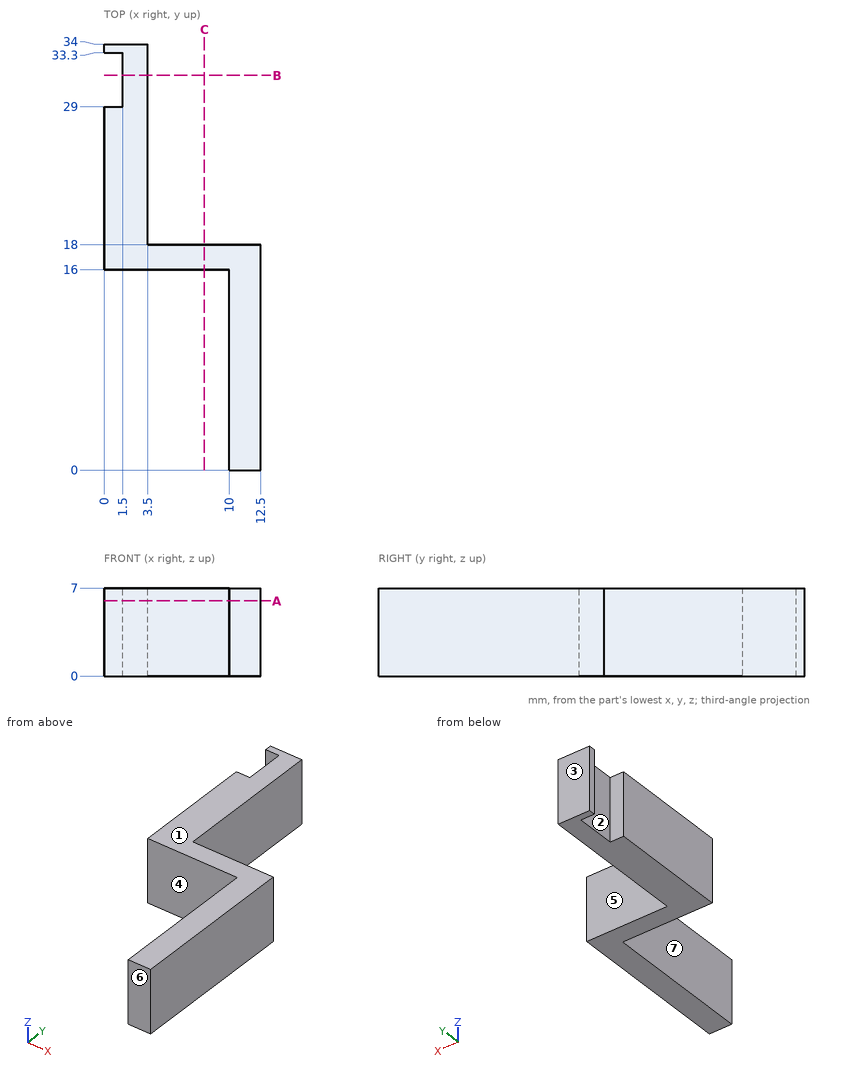
Can you work these out from the drawing? Everything is in mm from the part's minimum corner. A direction names the side the tool comes from. Round coordinates to 2 decimals unless told otherwise and drop trailing zeros. Write each loop counter-clockwise with the first axis right and the second up, starting at its lowest first coordinate (ties: lowest second). Pieces come first, ordered by that corner, then holes. Notation, with made-up numbers: M 63,28.25 L 119,28.25 A17 cw 119,36.25 Z; hole C -38,81.5 d2. An arc over 180 degrees is marked long. Use a Markdown table: item, result.
Item 1: I want a section at B-B (y = 31.5). List the corners of the cut face in (x, z) for me, and give its area (3 significant figures).
Found:
| item | result |
|---|---|
| outline | M 1.5,0 L 3.5,0 L 3.5,7 L 1.5,7 Z |
| area | 14.0 mm2 |
Item 2: I want a section at C-C (x = 8). List the corners of the cut face in (y, z) for me, and give its area (3 significant figures).
Found:
| item | result |
|---|---|
| outline | M 16,0 L 18,0 L 18,7 L 16,7 Z |
| area | 14.0 mm2 |
Item 3: For pin 1 Ø3.5 at (x, z) = (6.5, 3) entering from -Y; pin 2 Ø3.5 at (y, z) = (8, 2) entering from -X; pin 3 Ø3.5 at (x, z) = (8.5, 5) entering from +Y; pin 4 Ø4 at (x, y) = (7, 11) entering from -Z, each with a flat end and sliding along its axis, tell me the tip position at first contact or that it passes through.
Found:
| item | result |
|---|---|
| pin 1 | stops at y = 16 |
| pin 2 | stops at x = 10 |
| pin 3 | stops at y = 18 |
| pin 4 | passes through |
Item 4: We'd pull the mould along Y, two halves only. Please class the marked faces 1, 2, 3 and 4: released by +Y, released by -Y, zero draft, split by the parting line, or undercut.
Found:
| item | result |
|---|---|
| face 1 | zero draft |
| face 2 | undercut |
| face 3 | released by +Y |
| face 4 | released by -Y |
Item 5: I want a section at A-A (z = 6). List the corners of the cut face in (x, y) for me.
Found:
| item | result |
|---|---|
| outline | M 0,16 L 10,16 L 10,0 L 12.5,0 L 12.5,18 L 3.5,18 L 3.5,34 L 0,34 L 0,33.3 L 1.5,33.3 L 1.5,29 L 0,29 Z |
Item 6: If I drill on line 1 along Y through (x, z) = (1, 2); line 2 along Y through (x, z) = (6.5, 0.75); line 3 along X through (y, z) = (11, 3.75), over which ranges is the centre line in solid material (lowest first)? Write a range as [from, to].
Found:
| item | result |
|---|---|
| line 1 | y = [16, 29], [33.3, 34] |
| line 2 | y = [16, 18] |
| line 3 | x = [10, 12.5] |
Item 7: Which directions (+Z, -Z, +X, -X, +Y, -Y) give clear straight access to the entire face, cutting with the end or side of a thin tool? Please do the marked faces 5, 6 and 7.
Found:
| item | result |
|---|---|
| face 5 | +Z, -Z, +X, +Y |
| face 6 | +Z, -Z, +X, -X, -Y |
| face 7 | +Z, -Z, -X, -Y |
